Could you check a few things on this model? Use its own coordinates, in mm. Face numbers are marked on the shaded views. A direction names the side the tool comes from. Coordinates: 2 decimals unless noted, no trailing zeros. Order: outer loops, then holes, each group sorted by start corner. A loop starts at its lowest first (then second) coordinate and runs counter-clockwise, first axis right, second up. Notation, with made-up numbers: (75.5, -1.5) - (107.5, -1.5) arc R17 cw to (107.5, 21.5) - close; hole circle Ø9 at (18.25, 49.5). An arc over 180 degrees is marked (long way). One line per item, written item: value. Start each with the question number.
from build123d import *

# Parameters (mm, degrees)
BOSS_EXTRUDE1_DEPTH  = 20
SKETCH7_W            = 12
SKETCH7_H            = 20
SKETCH7_W_2          = 6.931673433
BOSS_EXTRUDE2_DEPTH  = 3
M3_CLEARANCE_HOLE2_D = 3.4
FILLET1_R            = 1


with BuildPart() as part:
    # Sketch3 → Boss-Extrude1 (new body)
    with BuildSketch(Plane.XY):
        Polygon((3, 0), (3, 15), (23, 15), (23, 0), (26, 0), (26, 18), (0, 18), (0, 0), align=None)
    extrude(amount=BOSS_EXTRUDE1_DEPTH)

    # Sketch7 → Boss-Extrude2 (add)
    with BuildSketch(Plane(origin=(0, 0, 0), x_dir=(1, 0, 0), z_dir=(0, 1, 0))):
        with Locations((-6, -10)):
            Rectangle(SKETCH7_W, SKETCH7_H)
        with Locations((29.465836717, -10)):
            Rectangle(SKETCH7_W_2, SKETCH7_H)
    extrude(amount=BOSS_EXTRUDE2_DEPTH)

    # M3 Clearance Hole2 (through all)
    with Locations(Plane(origin=(0, 3, 0), x_dir=(1, 0, 0), z_dir=(0, 1, 0))):
        with Locations((29.465836717, -10), (-6, -10)):
            Hole(M3_CLEARANCE_HOLE2_D / 2)

    # Fillet1
    fillet1_edges = [part.edges().sort_by_distance(p)[0] for p in [
        (0, 18, 10),
        (26, 18, 10),
        (23, 0, 10),
        (23, 15, 10),
        (3, 15, 10),
        (3, 0, 10),
        (32.931673433, 0, 10),
        (32.931673433, 3, 10),
        (-12, 0, 10),
        (0, 3, 10),
        (-12, 3, 10),
    ]]
    fillet(fillet1_edges, radius=FILLET1_R)


solid = part.part
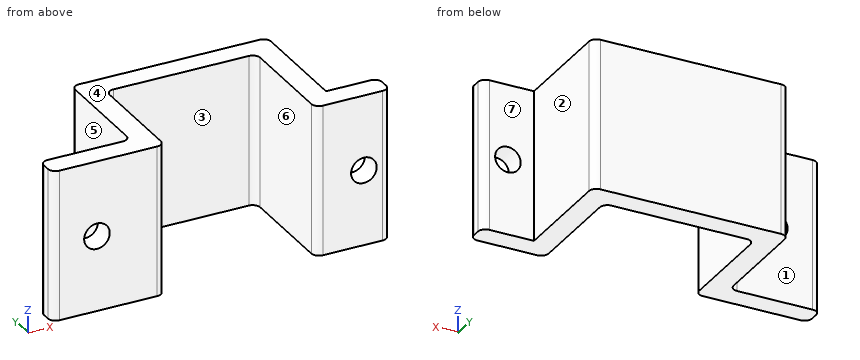
Q1. I want a section at B-B on y = 8.5. Please give me the cut outline in (x, z).
Q2. If I drill on L1, parallel to X at y = 2, z = 10; L2, parallel to X at y = 8, z = 4; L3, parallel to Z at x = -6, y = 1.25, over which ranges is the centre line in solid material (lowest first)?
Q3. I want a section at C-C on z = 10. State how many separate pieces and enclosed holes the cut face has, then the cut area to 3 significant figures.
Q4. I'm going to push flat-ended pins straight in: pin 1 (3 mm diameter, centred on y = 9, z = 8.5, fed in from +X); pin 2 (3 mm diameter, centred on x = -4.5, z = 11.5, fed in from +Y); pin 3 (5 mm diameter, centred on x = 18, y = 15, fed in from -Z); pin 4 (4 mm diameter, centred on y = 10.5, z = 9, fed in from -X). Where does each tip first touch, or does it pass through?
Q5. I want a section at D-D on z = 3.75. Please give me the cut outline in (x, y).
Q6. Which directions (+Z, -Z, +X, -X, +Y, -Y) give clear straight access to the entire face, cutting with the end or side of a thin tool? Please do the marked faces 1, 2, 3 and 4.
Q7. I want a section at A-A on x = -6. Please give me the cut outline in (y, z).
Q8. We'd pull the mould along X, two halves only. Please class the marked faces 5, 6 and 7: +X half, -X half, draft (parallel to the pull), parting line (faces both ways), or undercut.
Values follow:
1. outline: (0, 0) - (3, 0) - (3, 20) - (0, 20) - close; (23, 0) - (26, 0) - (26, 20) - (23, 20) - close
2. L1: x = -12 to -7.7, -4.3 to 3, 23 to 27.77, 31.17 to 32.93
2. L2: x = 0 to 3, 23 to 26
2. L3: z = 0 to 8.3, 11.7 to 20
3. separate pieces: 3
3. enclosed holes: 0
3. area: 203 mm^2
4. pin 1: stops at x = 26
4. pin 2: stops at y = 3
4. pin 3: stops at z = 0
4. pin 4: stops at x = 0
5. outline: (-12, 1) arc R1 ccw to (-11, 0) - (2, 0) arc R1 ccw to (3, 1) - (3, 14) arc R1 cw to (4, 15) - (22, 15) arc R1 cw to (23, 14) - (23, 1) arc R1 ccw to (24, 0) - (31.93, 0) arc R1 ccw to (32.93, 1) - (32.93, 2) arc R1 ccw to (31.93, 3) - (26, 3) - (26, 17) arc R1 ccw to (25, 18) - (1, 18) arc R1 ccw to (0, 17) - (0, 4) arc R1 cw to (-1, 3) - (-11, 3) arc R1 ccw to (-12, 2) - close
6. face 1: +Z, -Z, -X, +Y
6. face 2: +Z, -Z, +X, +Y
6. face 3: +Z, -Z, -Y
6. face 4: +Z, +X, -X, +Y, -Y
7. outline: (0, 0) - (3, 0) - (3, 8.3) - (0, 8.3) - close; (0, 11.7) - (3, 11.7) - (3, 20) - (0, 20) - close
8. face 5: -X half
8. face 6: undercut
8. face 7: draft
